from build123d import *

# Parameters (mm, degrees)
PAD_DEPTH       = 80
PAD_DEPTH_BACK  = 20
SKETCH001_R     = 2.6
SKETCH001_R_2   = 1.65
SKETCH001_R_3   = 0.5
POCKET_DEPTH    = 18.001
SKETCH002_W     = 66.71416
SKETCH002_H     = 42.248775
POCKET001_DEPTH = 13
SKETCH003_R     = 10.65
POCKET002_DEPTH = 30.4
SKETCH004_R     = 10.65
POCKET003_DEPTH = 30.4
POCKET004_DEPTH = 5
FILLET_R        = 5
FILLET001_R     = 1


with BuildPart() as part:
    # Sketch → Pad (new body, two sides)
    with BuildSketch(Plane.XZ) as pad_sk:
        with BuildLine():
            Line((-80, -18), (-80, -13))
            Line((-80, -13), (-20, -13))
            Line((-20, -13), (-20, 0))
            Line((-7, 0), (-20, 0))
            ThreePointArc((-7, 0), (0, -7), (7, 0))
            Line((7, 0), (20, 0))
            Line((20, 0), (20, -18))
            Line((20, -18), (-80, -18))
        make_face()
    extrude(amount=PAD_DEPTH)
    extrude(pad_sk.sketch, amount=-PAD_DEPTH_BACK)

    # Sketch001 → Pocket (cut, through all)
    with BuildSketch(Plane.XY):
        with Locations((-70, 10)):
            Circle(SKETCH001_R)
        with Locations((-30, 10)):
            Circle(SKETCH001_R)
        with Locations((10, 10)):
            Circle(SKETCH001_R)
        with Locations((-15, -5)):
            Circle(SKETCH001_R_2)
        with Locations((-15, -40)):
            Circle(SKETCH001_R_2)
        with Locations((-15, -75)):
            Circle(SKETCH001_R_2)
        with Locations((15, -5)):
            Circle(SKETCH001_R_2)
        with Locations((15, -40)):
            Circle(SKETCH001_R_2)
        with Locations((15, -75)):
            Circle(SKETCH001_R_2)
        with Locations((0, 20)):
            Circle(SKETCH001_R_3)
        Polygon((-80, 0), (-80, -80), (-20, -80), align=None)
    extrude(amount=-POCKET_DEPTH, mode=Mode.SUBTRACT)

    # Sketch002 → Pocket001 (cut)
    with BuildSketch(Plane.XY):
        with Locations((0, 21.124387)):
            Rectangle(SKETCH002_W, SKETCH002_H)
    extrude(amount=-POCKET001_DEPTH, mode=Mode.SUBTRACT)

    # Sketch003 (on DatumPlane) → Pocket002 (cut)
    with BuildSketch(Plane.XZ.offset(5)):
        Circle(SKETCH003_R)
    extrude(amount=POCKET002_DEPTH, mode=Mode.SUBTRACT)

    # Sketch004 (on DatumPlane) → Pocket003 (cut)
    with BuildSketch(Plane.XZ.offset(75)):
        Circle(SKETCH004_R)
    extrude(amount=-POCKET003_DEPTH, mode=Mode.SUBTRACT)

    # Sketch005 (on DatumPlane) → Pocket004 (cut)
    with BuildSketch(Plane.XY.offset(-18)):
        Polygon((-12.25, -6.587713), (-12.25, -3.412287), (-15, -1.824574), (-17.75, -3.412287), (-17.75, -6.587713), (-15, -8.175426), align=None)
        Polygon((17.75, -6.587713), (17.75, -3.412287), (15, -1.824574), (12.25, -3.412287), (12.25, -6.587713), (15, -8.175426), align=None)
        Polygon((-12.25, -41.587713), (-12.25, -38.412287), (-15, -36.824574), (-17.75, -38.412287), (-17.75, -41.587713), (-15, -43.175426), align=None)
        Polygon((17.75, -41.587713), (17.75, -38.412287), (15, -36.824574), (12.25, -38.412287), (12.25, -41.587713), (15, -43.175426), align=None)
        Polygon((-12.25, -76.587713), (-12.25, -73.412287), (-15, -71.824574), (-17.75, -73.412287), (-17.75, -76.587713), (-15, -78.175426), align=None)
        Polygon((17.75, -76.587713), (17.75, -73.412287), (15, -71.824574), (12.25, -73.412287), (12.25, -76.587713), (15, -78.175426), align=None)
    extrude(amount=POCKET004_DEPTH, mode=Mode.SUBTRACT)

    # Fillet
    fillet_edges = [part.edges().sort_by_distance(p)[0] for p in [
        (-80, 20, -15.5),
        (-80, 0, -15.5),
        (20, -80, -9),
        (20, 20, -15.5),
    ]]
    fillet(fillet_edges, radius=FILLET_R)

    # Fillet001
    fillet001_edges = [part.edges().sort_by_distance(p)[0] for p in [
        (-20, -40, -13),
        (0, 0, -13),
    ]]
    fillet(fillet001_edges, radius=FILLET001_R)


solid = part.part
Source: CAD feature listing. Evaluate the final solid. Frame: model axes, mm. A direction names the side the tool comes from. Round coordinates to 2 decimals unless told otherwise and drop trailing zeros. Loops run counter-clockwise (first coordinate to the right, second up) from the corner with the lowest first, then second, coordinate; pieces in that order, holes last. Notation, with made-up numbers: (15.5, 30.25) - (42.5, 30.25) arc R16 cw to (42.5, 56.25) - close; hole circle Ø5 at (-11, 30.5). An arc over 180 degrees is marked (long way). Write item = value, one per line. Start each with the question number.
(1) Pin query (flat end, axial travel): pin 1 (10 mm diameter, centred on x = -65, y = -21.5, fed in from +Z); pin 2 (5.5 mm diameter, centred on x = 4, z = -3, fed in from +Y); pin 3 (1.6 mm diameter, centred on y = -40, z = -15, fed in from -X). Return the tip coordinate at first contact, or that it passes through.
(2) Section query A-A, the plane y = -40. Output: boundary loops of the cut face in (x, z).
(3) Section query D-D, the plane x = -30. Output: boundary loops of the cut face in (y, z), plus the area to 3 significant figures.
(4) Pull-direction query (X, two-part tool) for faces 1 (the face through (-0.3, 0, -7.2)), 2 (the face through (12.25, -5, -16)), 3 (the face through (19, -78, -9)), 4 (the face through (-72.6, 10.1, -15.5)); classes: +X half, -X half, draft (parallel to the pull), parting line (faces both ways), or undercut.
(5) Ray query, line 1 along Y through (x, z) = (-15, -9.25); line 2 along Y through (x, z) = (9, -5); line 3 along Z through (x, y) = (11, 13). Return the intervals inside material, ascending. Write a range as from..to.
(6) Set-up query: faces 5 (the face through (16.524, -75.632, -6.409)), 6 (the face through (16.394, -2.63, -15.535)), 7 (the face through (0, -44.6, -8)). Return all of +Z, -Z, +X, -X, +Y, -Y with unobstructed straight access to the full face (end or side cutting, diameter ignored); none if empty.
(7) Section query B-B, the plane y = 10. Output: boundary loops of the cut face in (x, z).
(8) Section query C-C, the plane z = -3.25. State how many separate pieces and enclosed holes the cut face has, plus the area to 3 significant figures.
Conclusion:
q1.pin_1 = -13
q1.pin_2 = 0
q1.pin_3 = -50.6
q2.outline = (-50, -18) - (-17.75, -18) - (-17.75, -13) - (-16.65, -13) - (-16.65, 0) - (-20, 0) - (-20, -12) arc R1 cw to (-21, -13) - (-50, -13) - close; (-13.35, -13) - (-12.25, -13) - (-12.25, -18) - (12.25, -18) - (12.25, -13) - (13.35, -13) - (13.35, 0) - (7, 0) arc R7 cw to (-7, 0) - (-13.35, 0) - close; (16.65, -13) - (17.75, -13) - (17.75, -18) - (20, -18) - (20, 0) - (16.65, 0) - close
q3.outline = (-66.67, -18) - (7.4, -18) - (7.4, -13) - (-66.67, -13) - close; (12.6, -18) - (20, -18) - (20, -13) - (12.6, -13) - close
q3.area = 407 mm2
q4.face_1 = draft
q4.face_2 = undercut
q4.face_3 = +X half
q4.face_4 = undercut
q5.line_1 = -80..-76.65, -73.35..-41.65, -38.35..-6.65, -3.35..0
q5.line_2 = -80..-75, -44.6..-35.4, -5..0
q5.line_3 = -18..-13
q6.face_5 = +Z, -Z
q6.face_6 = -Z
q6.face_7 = +Z
q7.outline = (-80, -18) - (-72.6, -18) - (-72.6, -13) - (-80, -13) - close; (-67.4, -18) - (-32.6, -18) - (-32.6, -13) - (-67.4, -13) - close; (-27.4, -18) - (7.4, -18) - (7.4, -13) - (-27.4, -13) - close; (12.6, -18) - (20, -18) - (20, -13) - (12.6, -13) - close
q8.separate_pieces = 2
q8.enclosed_holes = 6
q8.area = 1,670 mm2
